from build123d import *

# Parameters (mm, degrees)
F0_W     = 24
F0_H     = 16
F1_DEPTH = 10
F2_T     = -1.5
F3_R     = 2.425
F4_DEPTH = 1.6
F5_R     = 2.925
F6_DEPTH = 10


with BuildPart() as f1:
    # F0 (on Top) → F1 (new body)
    with BuildSketch(Plane.XY):
        Rectangle(F0_W, F0_H)
    extrude(amount=F1_DEPTH)

    # F2
    f2_openings = [f1.faces().sort_by_distance(p)[0] for p in [
        (0, 0, 0),
    ]]
    offset(amount=F2_T, openings=f2_openings)

    # F3 (on face) → F4 (join)
    with BuildSketch(Plane.XY.offset(10)):
        with Locations((-8, -4)):
            Circle(F3_R)
        with Locations((-8, 4)):
            Circle(F3_R)
        with Locations((0, -4)):
            Circle(F3_R)
        with Locations((0, 4)):
            Circle(F3_R)
        with Locations((8, -4)):
            Circle(F3_R)
        with Locations((8, 4)):
            Circle(F3_R)
    extrude(amount=F4_DEPTH)

    # F5 (on face) → F6 (join)
    with BuildSketch(Plane.XY.offset(10)):
        with Locations((-4, 0)):
            Circle(F5_R)
        with Locations((4, 0)):
            Circle(F5_R)
    extrude(amount=-F6_DEPTH)


solid = f1.part
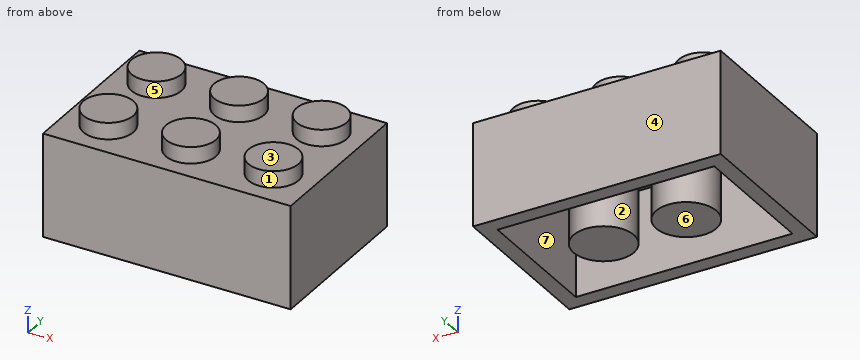
The listing builds one solid part. Answer for the finished solid, in the listing's coordinates (mm). Face numbers are marked on the shaded views. A direction names the side the tool comes from. Round coordinates to 2 decimals unless told otherwise and drop trailing zeros. Order: outer loops, then holes, each group sorted by start corner. A loop starts at its lowest first (then second) coordinate and runs counter-clockwise, first axis right, second up. Notation, with made-up numbers: (13.5, -20.5) -> (68.5, -20.5) arc R31 cw to (68.5, 15.5) -> close; hole circle Ø5 at (15, -28.5). An arc over 180 degrees is marked (long way). Write each question's results on one line, items separated by ' | '. Start each with the question number.
Q1. The mould has two halves that part along Y. Classify the marked faces 4, 5, 6 and 7: pulls with the +Y half, pulls with the -Y half, needs draft (parallel to the pull), parting line crosses it, or undercut.
Q2. Find section A-A (z = 6). Determine the outline of the cut face in (x, y) (3 decimals).
Q3. Find section D-D (x = -4). Determine the outline of the cut face in (y, z) (3 decimals), then the cut area to 3 significant figures.
Q4. Find section B-B (x = -8). Determine the outline of the cut face in (y, z) (3 decimals).
Q5. Straight lines are drawn through the part: probe 1 along X at (y, z) = (-5.5, 8); probe 2 along Y at (x, z) = (9.5, 6.25); probe 3 along X at (y, z) = (-1, 1.75). For each, find the intervals that lie inside material, in ascending order. Write a range as from..to.
Q6. Which of the six approach directions +Z, -Z, +X, -X, +Y, -Y give full straight-line access (tool end or side, diameter ignored) to the marked faces 1, 2 and 3?
Q7. Find section C-C (y = 0). Determine the outline of the cut face in (x, z) (3 decimals).
Worked answers:
1) face 4: pulls with the +Y half | face 5: undercut | face 6: needs draft | face 7: undercut
2) outline: (-12, -8) -> (12, -8) -> (12, 8) -> (-12, 8) -> close; circle Ø5.85 at (-4, 0); circle Ø5.85 at (4, 0); hole (-10.5, -6.5) -> (10.5, -6.5) -> (10.5, 6.5) -> (-10.5, 6.5) -> close
3) outline: (-8, 0) -> (-6.5, 0) -> (-6.5, 8.5) -> (-2.925, 8.5) -> (-2.925, 0) -> (2.925, 0) -> (2.925, 8.5) -> (6.5, 8.5) -> (6.5, 0) -> (8, 0) -> (8, 10) -> (-8, 10) -> close | area: 99.2 mm2
4) outline: (-8, 0) -> (-6.5, 0) -> (-6.5, 8.5) -> (6.5, 8.5) -> (6.5, 0) -> (8, 0) -> (8, 10) -> (6.425, 10) -> (6.425, 11.6) -> (1.575, 11.6) -> (1.575, 10) -> (-1.575, 10) -> (-1.575, 11.6) -> (-6.425, 11.6) -> (-6.425, 10) -> (-8, 10) -> close
5) probe 1: x = -12..-10.5, 10.5..12 | probe 2: y = -8..-6.5, 6.5..8 | probe 3: x = -12..-10.5, -6.75..-1.25, 1.25..6.75, 10.5..12
6) face 1: +Z | face 2: -Z | face 3: +Z, +X, -X, +Y, -Y
7) outline: (-12, 0) -> (-10.5, 0) -> (-10.5, 8.5) -> (-6.925, 8.5) -> (-6.925, 0) -> (-1.075, 0) -> (-1.075, 8.5) -> (1.075, 8.5) -> (1.075, 0) -> (6.925, 0) -> (6.925, 8.5) -> (10.5, 8.5) -> (10.5, 0) -> (12, 0) -> (12, 10) -> (-12, 10) -> close
